from build123d import *

# Parameters (mm, degrees)
SKETCH_1_W             = 34
SKETCH_1_H             = 60
EXTRUDE_443_DEPTH      = 12
SKETCH_2_R             = 2.1
CUT_EXTRUDE_710_DEPTH  = 13
SKETCH_3_R             = 12.5
CUT_EXTRUDE_893_DEPTH  = 9
SKETCH_4_R             = 6.55
CUT_EXTRUDE_999_DEPTH  = 4
SKETCH_5_R             = 1.55
CUT_EXTRUDE_1168_DEPTH = 4
FILLET_4_R             = 4
SKETCH_6_R             = 2.1
SKETCH_6_R_2           = 1.5
EXTRUDE_1_DEPTH        = 12


with BuildPart() as part:
    # 草图1 → Extrude 443 (new body)
    with BuildSketch(Plane(origin=(0, 0, 0), x_dir=(1, 0, 0), z_dir=(0, 1, 0))):
        Rectangle(SKETCH_1_W, SKETCH_1_H)
    extrude(amount=EXTRUDE_443_DEPTH)

    # 草图2 → Cut-Extrude 710 (cut, through all)
    with BuildSketch(Plane(origin=(0, 12, 0), x_dir=(1, 0, 0), z_dir=(0, 1, 0))):
        with Locations((-12, -25)):
            Circle(SKETCH_2_R)
        with Locations((12, -25)):
            Circle(SKETCH_2_R)
    extrude(amount=-CUT_EXTRUDE_710_DEPTH, mode=Mode.SUBTRACT)

    # 草图3 → Cut-Extrude 893 (cut)
    with BuildSketch(Plane(origin=(0, 12, 0), x_dir=(1, 0, 0), z_dir=(0, 1, 0))):
        with Locations((0, 16)):
            Circle(SKETCH_3_R)
    extrude(amount=-CUT_EXTRUDE_893_DEPTH, mode=Mode.SUBTRACT)

    # 草图4 → Cut-Extrude 999 (cut, through all)
    with BuildSketch(Plane(origin=(0, 3, 0), x_dir=(1, 0, 0), z_dir=(0, 1, 0))):
        with Locations((0, 16)):
            Circle(SKETCH_4_R)
    extrude(amount=-CUT_EXTRUDE_999_DEPTH, mode=Mode.SUBTRACT)

    # 草图5 → Cut-Extrude 1168 (cut, through all)
    with BuildSketch(Plane(origin=(0, 3, 0), x_dir=(1, 0, 0), z_dir=(0, 1, 0))):
        with Locations((0, 25.5)):
            Circle(SKETCH_5_R)
        with Locations((8.227241336, 11.25)):
            Circle(SKETCH_5_R)
        with Locations((-8.227241336, 11.25)):
            Circle(SKETCH_5_R)
    extrude(amount=-CUT_EXTRUDE_1168_DEPTH, mode=Mode.SUBTRACT)

    # 圆角4
    fillet_4_edges = [part.edges().sort_by_distance(p)[0] for p in [
        (17, 6, 30),
        (-17, 6, 30),
        (-17, 6, -30),
        (17, 6, -30),
    ]]
    fillet(fillet_4_edges, radius=FILLET_4_R)

    # 草图6 → 凸台-拉伸1 (add)
    with BuildSketch(Plane(origin=(0, 12, 0), x_dir=(1, 0, 0), z_dir=(0, 1, 0))):
        with Locations((-12, -25)):
            Circle(SKETCH_6_R)
        with Locations((-12, -25)):
            Circle(SKETCH_6_R_2, mode=Mode.SUBTRACT)
        with Locations((12, -25)):
            Circle(SKETCH_6_R)
        with Locations((12, -25)):
            Circle(SKETCH_6_R_2, mode=Mode.SUBTRACT)
    extrude(amount=-EXTRUDE_1_DEPTH)


solid = part.part
Work out the finished part from the listing and answer in its coordinate system (mm). Coordinates: 2 decimals unless noted, no trailing zeros. Order: outer loops, then holes, each group sorted by start corner. A loop starts at its lowest first (then second) coordinate and runs counter-clockwise, first axis right, second up. Notation, with made-up numbers: (2.5, 79.25) - (57.5, 79.25) arc R9 ccw to (57.5, 83.25) - close; hole circle Ø1 at (78, 74.5). An arc over 180 degrees is marked (long way). Put each result on its own line as item: value. Start each with the question number.
1) Find section D-D (x = -4). Give the vertices of the cut face in (y, z), plus the area to 3 significant figures.
2) Find section C-C (y = 4). Give the vertices of the cut face in (x, z).
3) Find section A-A (x = 0). Give the vertices of the cut face in (y, z).
4) For a pull along Z with two mould halves and no side action, classify faces 1 (the cylindrical face through (5.77, 7.56, -4.91)), 2 (the flat face through (5, 3, -11)), 3 (the flat face through (0, 6, -30)), 4 (the flat face through (0, 6, 30)) as released by +Z, released by -Z, zero draft, split by the parting line, or undercut.
5) Find the intervals of material crossed by line 1 (X direction, y = 1, z = 25); line 2 (Z direction, x = 0, y = 1.45); line 3 (Z direction, x = 0, y = 7.5), in increasing order. Write a range as from..to.
6) Find section B-B (z = 25). Give the vertices of the cut face in (x, y).
7) Flat-ended cylindrical pins translate along their axes: pin 1 (3.5 mm diameter, centred on x = -12, z = 25, fed in from +Y); pin 2 (5 mm diameter, centred on x = 8.23, z = -11.25, fed in from +Y). Find the tip coordinate at first contact, or state that the pin passes through.
Results list:
1. outline: (0, -30) - (12, -30) - (12, -27.84) - (3, -27.84) - (3, -21.19) - (0, -21.19) - close; (0, -10.81) - (3, -10.81) - (3, -4.16) - (12, -4.16) - (12, 30) - (0, 30) - close
1. area: 476 mm^2
2. outline: (-17, -26) arc R4 ccw to (-13, -30) - (13, -30) arc R4 ccw to (17, -26) - (17, 26) arc R4 ccw to (13, 30) - (-13, 30) arc R4 ccw to (-17, 26) - close; hole circle Ø3 at (-12, 25); hole circle Ø25 at (0, -16); hole circle Ø3 at (12, 25)
3. outline: (0, -30) - (12, -30) - (12, -28.5) - (3, -28.5) - (3, -27.05) - (0, -27.05) - close; (0, -23.95) - (3, -23.95) - (3, -22.55) - (0, -22.55) - close; (0, -9.45) - (3, -9.45) - (3, -3.5) - (12, -3.5) - (12, 30) - (0, 30) - close
4. face 1: undercut
4. face 2: undercut
4. face 3: released by -Z
4. face 4: released by +Z
5. line 1: x = -17..-13.5, -10.5..10.5, 13.5..17
5. line 2: z = -30..-27.05, -23.95..-22.55, -9.45..30
5. line 3: z = -30..-28.5, -3.5..30
6. outline: (-17, 0) - (-13.5, 0) - (-13.5, 12) - (-17, 12) - close; (-10.5, 0) - (10.5, 0) - (10.5, 12) - (-10.5, 12) - close; (13.5, 0) - (17, 0) - (17, 12) - (13.5, 12) - close
7. pin 1: stops at y = 12
7. pin 2: stops at y = 3
